For this review, take the finished solid that the model builds, in its own axes (mm). A direction names the side the tool comes from. Give positions to 0.01 mm unless a question says otherwise; leave off trailing zeros. Order: outer loops, then holes, each group sorted by start corner. A loop starts at its lowest first (then second) coordinate and runs counter-clockwise, first axis right, second up.
Item 1: Machinability: for faces 1 (the flat face through (-21, 3, -53)), 2 (the flat face through (-40.5, 7, -43)), 3 (the flat face through (-28, 3, -33)), which of the approach directions +Z, -Z, +X, -X, +Y, -Y give a long, thin tool a straight path to every point of the face, cutting with its end or side? Answer none if there is none.
Item 2: For P1, Ø12, axis at x = -41, z = -34, coming from the -Y side; P2, Ø2.5, axis at y = 6.75, z = -47.75, coming from the +X side; P3, Ø1.2, axis at y = 1, z = -5, coming from the -X side, all flat-tipped, find the tip position at first contact; note any pin that passes through.
Item 3: The part is to be moulded in two halves that separate along Y. For faces 4 (the flat face through (-15, 0, -36)), 5 (the cylindrical face through (-43.54, 7.08, -37.2)), 6 (the cylindrical face through (2.8, 2, -0.1)), say which applies: released by +Y, released by -Y, zero draft, split by the parting line, or undercut.
Item 4: Consider section A-A (z = -38.25). Give the boundary of the cut face in (x, y).
Item 5: For probe 1 along Z at (x, y) = (-43.8, 6.75); probe 2 along Z at (x, y) = (0, 2.2); probe 3 along Y at (x, z) = (-44.1, -47.75), list the stretches that pass through material, from the lowest coordinate up.
Item 6: Consider section B-B (x = 0). Give the boundary of the cut face in (y, z), plus the area to 3 significant figures.
Item 7: Consider section D-D (y = 6.75). Give the boundary of the cut face in (x, z), plus the area to 3 significant figures.
Item 8: Consider section C-C (y = 1.5). Give the boundary of the cut face in (x, z).
Autodesk Inventor part; units mm, degrees
ref_plane "YZ Plane" through (0, 0, 0) normal (1, 0, 0) x (0, 1, 0)
ref_plane "XZ Plane" through (0, 0, 0) normal (0, 1, 0) x (-1, 0, 0)
ref_plane "XY Plane" through (0, 0, 0) normal (0, 0, 1) x (1, 0, 0)
sketch "Sketch1" plane through (0, 0, 0) normal (0, 1, 0) x (-1, 0, 0)
  line L0 (0, 0) -> (40.5, 0)
  line L1 (40.5, 0) -> (40.5, -47)
  line L2 (40.5, -47) -> (0, -47)
  line L3 (0, -47) -> (0, 0)
  circle A0 centre (0, 0) radius 2.8
  circle A1 centre (0, -47) radius 2.8
  line L4 (0, 0) -> (-6, 0)
  line L5 (-6, 0) -> (-6, 6)
  line L6 (0, -47) -> (-6, -47)
  line L7 (-6, -47) -> (-6, -53)
  line L8 (-6, -53) -> (40.5, -53)
  line L9 (40.5, -53) -> (-6, -53)
  line L10 (-6, -53) -> (-6, 6)
  line L11 (-6, 6) -> (40.5, 6)
  line L12 (40.5, 6) -> (40.5, -53)
  line L13 (40.5, 6) -> (46.5, 6)
  line L14 (46.5, 6) -> (46.5, -53)
  line L15 (46.5, -53) -> (40.5, -53)
  line L16 (40.5, -53) -> (40.5, 6)
  dimension "d0" = 40.5
  dimension "d1" = 47
  dimension "d2" = 5.6
  dimension "d3" = 5.6
  dimension "d4" = 6
  dimension "d5" = 6
  dimension "d6" = 6
  dimension "d7" = 6
  dimension "d8" = 6
extrude "Extrusion1" add sketch "Sketch1" along normal blind 4 contours A0 L4 L5 L11 L12 L0 | L0 L1 L2 A1 L3 A0 | L3 A1 L6 L10 L4 A0 | L12 L13 L14 L15 L1 | L12 L8 L7 L6 A1 L2
sketch "Sketch3" plane through (-46.5, 0, -53) normal (-1, 0, 0) x (0, 0, 1)
  line L0 (0, 0) -> (0, 4)
  line L1 (0, 4) -> (20, 4)
  line L2 (20, 4) -> (20, 9)
  line L3 (20, 9) -> (0, 9)
  line L4 (0, 9) -> (0, 4)
  point P0 (53, 0)
  dimension "d11" = 20
  dimension "d12" = 5
extrude "Extrusion2" add sketch "Sketch3" against normal blind 6
sketch "Sketch4" plane through (0, 4, 0) normal (0, 1, 0) x (1, 0, 0)
  line L0 (-46.5, -6) -> (6, -6)
  line L1 (-46.5, -6) -> (-8.5, -6)
  line L2 (-8.5, -6) -> (-8.5, 36)
  line L3 (-8.5, 36) -> (-46.5, 36)
  line L4 (-46.5, 36) -> (-46.5, -6)
  point P0 (0, 0)
  dimension "d15" = 38
  dimension "d16" = 42
extrude "Extrusion3" cut sketch "Sketch4" against normal blind 6
sketch "Sketch5" plane through (-46.5, 9, -53) normal (-1, 0, 0) x (0, 0, 1)
  line L0 (20, 0) -> (0, 0)
  line L1 (10, 0) -> (5.25, 0)
  line L2 (5.25, 0) -> (5.25, 2.25)
  line L3 (5.25, 0) -> (5.25, -2.25)
  line L4 (5.25, -2.25) -> (14.75, -2.25)
  circle A0 centre (5.25, -2.25) radius 1.1
  circle A1 centre (14.75, -2.25) radius 1.1
  point P0 (53, -9)
  dimension "d19" = 4.75
  dimension "d20" = 2.25
  dimension "d21" = 90
  dimension "d22" = 2.25
  dimension "d23" = 9.5
  dimension "d24" = 2.2
  dimension "d25" = 2.2
extrude "Extrusion4" cut sketch "Sketch5" against normal blind 6
sketch "Sketch6" plane through (0, 4, 0) normal (0, -1, 0) x (1, 0, 0)
  line L0 (-46.5, -36) -> (-46.5, -33)
  line L1 (-8.5, -36) -> (-8.5, 6)
  line L2 (-46.5, -33) -> (-8.5, -33)
  line L3 (-8.5, -33) -> (-8.5, -36)
  line L4 (-8.5, -36) -> (-46.5, -36)
  line L5 (-46.5, -36) -> (-46.5, -33)
  point P0 (0, 0)
extrude "Extrusion5" add sketch "Sketch6" along normal blind 4
properties part number "limit_switch_lower_mount"
Resolved:
1. face 1: -Z, +X, -X, +Y, -Y
1. face 2: +Z, -Z, +X, +Y
1. face 3: +Z, -X, +Y, -Y
2. P1: stops at y = 0
2. P2: stops at x = -40.5
2. P3: stops at x = -8.5
3. face 4: released by -Y
3. face 5: undercut
3. face 6: zero draft
4. outline: (-46.5, 0) - (6, 0) - (6, 4) - (-40.5, 4) - (-40.5, 5.65) - (-46.5, 5.65) - close; (-46.5, 7.85) - (-40.5, 7.85) - (-40.5, 9) - (-46.5, 9) - close
5. probe 1: z = -53 to -48.85, -46.65 to -39.35, -37.15 to -33
5. probe 2: z = -53 to -49.8, -44.2 to -2.8, 2.8 to 6
5. probe 3: y = 0 to 5.65, 7.85 to 9
6. outline: (0, -53) - (4, -53) - (4, -49.8) - (0, -49.8) - close; (0, -44.2) - (4, -44.2) - (4, -2.8) - (0, -2.8) - close; (0, 2.8) - (4, 2.8) - (4, 6) - (0, 6) - close
6. area: 191 mm2
7. outline: (-46.5, -53) - (-40.5, -53) - (-40.5, -48.85) - (-46.5, -48.85) - close; (-46.5, -46.65) - (-40.5, -46.65) - (-40.5, -39.35) - (-46.5, -39.35) - close; (-46.5, -37.15) - (-40.5, -37.15) - (-40.5, -33) - (-46.5, -33) - close
7. area: 93.6 mm2
8. outline: (-46.5, -53) - (6, -53) - (6, 6) - (-8.5, 6) - (-8.5, -33) - (-46.5, -33) - close; hole circle Ø5.6 at (0, -47); hole circle Ø5.6 at (0, 0)
